Here's how the part is built. I have some questions about the finished solid (model axes, mm). Face numbers are marked on the shaded views. A direction names the side the tool comes from. Round coordinates to 2 decimals unless told otherwise and drop trailing zeros. Write each loop counter-clockwise with the first axis right and the second up, starting at its lowest first coordinate (ties: lowest second). Pieces come first, ordered by that corner, then holes. Notation, with made-up numbers: M -7.75,-32 L 20.25,-32 A14 cw 20.25,-12 Z; hole C 56.5,47.25 d5. An arc over 180 degrees is marked long. Write item = value, one per line. Start each with the question number.
(1) I need wall thicknesses on line 1 along X through (y, z) = (34, 38); line 2 along X through (y, z) = (-4, 9); line 3 along X through (y, z) = (-7.5, 22). Which ranges of each line are inside material? Lowest first, please.
(2) Will these pins go through, and if not, where does the flat tip stop? pin 1 Ø1.6 at (x, z) = (-6.5, -9) entering from -Y; pin 2 Ø3.5 at (x, z) = (-69, 12) entering from -Y; pin 3 Ø8 at (x, z) = (-47, 62) entering from -Y; pin 4 Ø11 at (y, z) = (8.5, -4.5) entering from -X.
(3) I want a section at A-A (z = 147.5). List the corners of the cut face in (x, y) for me.
(4) On a 3-axis mill with a long thin cutter (end or side, diameter ignored), from which of +Z, -Z, +X, -X, +Y, -Y can I reach the whole of each face in a straight line? I mean the marked faces 1 and 2. Say none if no direction works.
(5) I want a section at B-B (y = 44.5). List the corners of the cut face in (x, z) for me.
(6) I want a section at D-D (x = 31). List the corners of the cut face in (y, z) for me.
(7) I want a section at C-C (x = 75.5). List the corners of the cut face in (y, z) for me, and give its area (3 significant figures).
```python
from build123d import *

# Parameters (mm, degrees)
EXTRUDE_1_DEPTH          = 3
EXTRUDE_2_DEPTH          = 121.210911
SKETCH_3_W               = 47.605950515
SKETCH_3_H               = 3
CUT_EXTRUDE_1_DEPTH      = 99
SKETCH_5_W               = 185.441878516
SKETCH_5_H               = 108.742952173
CUT_EXTRUDE_2_DEPTH      = 1.5
SKETCH_6_W               = 175.21190103
SKETCH_6_H               = 36.65
EXTRUDE_3_DEPTH          = 7.2
SHELL_START              = 5.5
SHELL_1_DEPTH            = 114.710911355
SHELL_START_2            = 2.5
SHELL_1_2_OUTLINE_W      = 170.21190103
SHELL_1_2_OUTLINE_H      = 34.15
SHELL_1_2_DEPTH          = 124.910911355
SHELL_1_3_DEPTH          = 20.210911355
SHELL_1_4_DEPTH          = 17.210911355
SKETCH_7_W               = 170.21190103
SKETCH_7_H               = 34.15
CUT_EXTRUDE_3_DEPTH      = 7.2
SKETCH_8_W               = 2.5
SKETCH_8_H               = 36.65
EXTRUDE_4_DEPTH          = 45
CUT_EXTRUDE_4_DEPTH      = 261.975558395
SKETCH_10_W              = 2.5
SKETCH_10_H              = 2.880985124
EXTRUDE_5_DEPTH          = 124.689092
SKETCH_11_W              = 36.523943303
SKETCH_11_H              = 3
EXTRUDE_6_DEPTH          = 15
SKETCH_12_W              = 36.475357481
SKETCH_12_H              = 3.054288943
EXTRUDE_7_DEPTH          = 15
FILLET_1_R               = 25
SKETCH_13_W              = 43.927566906
SKETCH_13_H              = 9.945864205
EXTRUDE_8_DEPTH          = 8
CUT_EXTRUDE_5_DEPTH      = 219.603325421
SKETCH_15_W              = 43.927566906
SKETCH_15_H              = 9.945864205
EXTRUDE_9_DEPTH          = 2
SKETCH_17_W              = 27.673413216
SKETCH_17_H              = 3
EXTRUDE_10_DEPTH         = 12
RIB_1_REACH              = 263.024
SKETCH_18_WALL_W         = 539.179228978
SKETCH_18_WALL_H         = 3
MIRROR_5_COPY_1_REACH    = 263.024
MIRROR_5_COPY_1_SKETCH_W = 539.179228978
MIRROR_5_COPY_1_SKETCH_H = 3
RIB_2_REACH              = 175.005
SKETCH_19_WALL_W         = 366.464948776
SKETCH_19_WALL_H         = 3
MIRROR_7_COPY_1_REACH    = 175.005
MIRROR_7_COPY_1_SKETCH_W = 366.464948776
MIRROR_7_COPY_1_SKETCH_H = 3
RIB_3_REACH              = 153.018
SKETCH_20_WALL_W         = 334.972416452
SKETCH_20_WALL_H         = 3
EXTRUDE_11_DEPTH         = 20.47
CUT_EXTRUDE_6_DEPTH      = 264.412642976


# Read off the part's stored shape, not the designer's step: 抽壳1
with BuildPart() as part:
    # 草图1 → 凸台-拉伸1 (new body)
    with BuildSketch(Plane.XY):
        Polygon((-100, 0), (-60, 0), (-60, -3.3), (-100, -3.3), (-100, -23.3), (100, -23.3), (100, -3.3), (60, -3.3), (60, 0), (100, 0), (100, 39.5), (-100, 39.5), align=None)
    extrude(amount=EXTRUDE_1_DEPTH)

    # 草图2 → 凸台-拉伸2 (add)
    with BuildSketch(Plane.XY.offset(3)):
        Polygon((40, -48.15), (-40, -48.15), (-40, -0.15), (-87.605950515, -0.030985124), (-87.605950515, 39.5), (87.605950515, 39.5), (87.605950515, -0.030985124), (40, -0.15), align=None)
    extrude(amount=EXTRUDE_2_DEPTH)

    # 草图3 → 切除-拉伸1 (cut)
    with BuildSketch(Plane.XY.offset(124.210911355)):
        with Locations((63.802975258, 1.35)):
            Rectangle(SKETCH_3_W, SKETCH_3_H)
        with Locations((-63.802975258, 1.35)):
            Rectangle(SKETCH_3_W, SKETCH_3_H)
    extrude(amount=-CUT_EXTRUDE_1_DEPTH, mode=Mode.SUBTRACT)

    # 草图5 → 切除-拉伸2 (cut)
    with BuildSketch(Plane.XY.offset(124.210911355)):
        with Locations((-1.343781728, 1.77370169)):
            Rectangle(SKETCH_5_W, SKETCH_5_H)
    extrude(amount=-CUT_EXTRUDE_2_DEPTH, mode=Mode.SUBTRACT)

    # 草图6 → 凸台-拉伸3 (add)
    with BuildSketch(Plane.XY.offset(122.710911355)):
        with Locations((0, 21.175)):
            Rectangle(SKETCH_6_W, SKETCH_6_H)
    extrude(amount=EXTRUDE_3_DEPTH)

    # 抽壳1 outline → 抽壳1 (cut)
    with BuildSketch(Plane.XY.offset(SHELL_START)):
        Polygon((-85.105950515, 39.5), (-85.105950515, 5.35), (-37.5, 5.35), (-37.5, -45.65), (37.5, -45.65), (37.5, 5.35), (85.105950515, 5.35), (85.105950515, 39.5), align=None)
    extrude(amount=SHELL_1_DEPTH, mode=Mode.SUBTRACT)

    # Shell 1 2 outline → Shell 1 2 (cut)
    with BuildSketch(Plane.XY.offset(SHELL_START_2)):
        with Locations((0, 22.425)):
            Rectangle(SHELL_1_2_OUTLINE_W, SHELL_1_2_OUTLINE_H)
    extrude(amount=SHELL_1_2_DEPTH, mode=Mode.SUBTRACT)

    # Shell 1 3 outline → Shell 1 3 (cut)
    with BuildSketch(Plane.XY.offset(SHELL_START_2)):
        Polygon((-85.105950515, 5.35), (-85.105950515, 2.5), (-57.5, 2.5), (-57.5, 2.393757812), (-37.5, 2.343757812), (-37.5, -20.8), (37.5, -20.8), (37.5, 2.343757812), (57.5, 2.393757812), (57.5, 2.5), (85.105950515, 2.5), (85.105950515, 5.35), align=None)
    extrude(amount=SHELL_1_3_DEPTH, mode=Mode.SUBTRACT)

    # Shell 1 4 outline → Shell 1 4 (cut)
    with BuildSketch(Plane.XY.offset(SHELL_START)):
        Polygon((-85.105950515, 2.5), (-85.105950515, 2.462772689), (-57.5, 2.393757812), (-57.5, 2.5), align=None)
        Polygon((85.105950515, 2.462772689), (85.105950515, 2.5), (57.5, 2.5), (57.5, 2.393757812), align=None)
    extrude(amount=SHELL_1_4_DEPTH, mode=Mode.SUBTRACT)

    # 草图7 → 切除-拉伸3 (cut)
    with BuildSketch(Plane.XY.offset(129.910911355)):
        with Locations((0, 22.425)):
            Rectangle(SKETCH_7_W, SKETCH_7_H)
    extrude(amount=-CUT_EXTRUDE_3_DEPTH, mode=Mode.SUBTRACT)

    # 草图8 → 凸台-拉伸4 (add)
    with BuildSketch(Plane.XY.offset(129.910911355)):
        with Locations((86.355950515, 21.175)):
            Rectangle(SKETCH_8_W, SKETCH_8_H)
    extrude_4 = extrude(amount=EXTRUDE_4_DEPTH)

    # 镜向1: 凸台-拉伸4 across plane
    add(extrude_4.mirror(Plane(origin=(0, 0, 0), x_dir=(0, 0, 1), z_dir=(1, 0, 0))))

    # 草图9 → 切除-拉伸4 (cut, through all)
    with BuildSketch(Plane(origin=(87.605950515, 0, 0), x_dir=(0, 0, -1), z_dir=(1, 0, 0))):
        with BuildLine():
            ThreePointArc((-153.435169701, 14.152379613), (-157.269646082, 19.530454036), (-163.545332043, 21.590225708))
            Line((-163.545332043, 21.590225708), (-164.318099098, 21.561993734))
            Line((-164.318099098, 21.561993734), (-174.910911355, 21.175))
            Line((-174.910911355, 21.175), (-174.910911355, 2.85))
            Line((-174.910911355, 2.85), (-149.900003415, 2.85))
            Line((-149.900003415, 2.85), (-153.435169701, 14.152379613))
        make_face()
    extrude(amount=-CUT_EXTRUDE_4_DEPTH, mode=Mode.SUBTRACT)

    # 草图10 → 凸台-拉伸5 (add)
    with BuildSketch(Plane.XY.offset(25.210911355)):
        with Locations((86.355950515, 1.409507438)):
            Rectangle(SKETCH_10_W, SKETCH_10_H)
        with Locations((-86.355950515, 1.409507438)):
            Rectangle(SKETCH_10_W, SKETCH_10_H)
    extrude(amount=EXTRUDE_5_DEPTH)

    # 草图11 → 凸台-拉伸6 (add)
    with BuildSketch(Plane(origin=(40, 0, 0), x_dir=(0, 0, -1), z_dir=(1, 0, 0))):
        with Locations((-104.448939704, -4.8)):
            Rectangle(SKETCH_11_W, SKETCH_11_H)
    extrude_6 = extrude(amount=EXTRUDE_6_DEPTH)

    # 镜向2: 凸台-拉伸6 across plane
    add(extrude_6.mirror(Plane(origin=(0, 0, 0), x_dir=(0, 0, 1), z_dir=(1, 0, 0))))

    # 草图12 → 凸台-拉伸7 (add)
    with BuildSketch(Plane(origin=(40, 0, 0), x_dir=(0, 0, -1), z_dir=(1, 0, 0))):
        with Locations((-104.525351124, 1.496159348)):
            Rectangle(SKETCH_12_W, SKETCH_12_H)
    extrude_7 = extrude(amount=EXTRUDE_7_DEPTH)

    # 镜向3: 凸台-拉伸7 across plane
    add(extrude_7.mirror(Plane(origin=(0, 0, 0), x_dir=(0, 0, 1), z_dir=(1, 0, 0))))

    # 圆角1
    fillet_1_edges = [part.edges().sort_by_distance(p)[0] for p in [
        (0, -48.15, 122.710911355),
        (0, -45.65, 120.210911355),
    ]]
    fillet(fillet_1_edges, radius=FILLET_1_R)

    # 草图13 → 凸台-拉伸8 (add)
    with BuildSketch(Plane(origin=(0, 0, 0), x_dir=(-1, 0, 0), z_dir=(0, 0, -1))):
        with Locations((0, 10.69739906)):
            Rectangle(SKETCH_13_W, SKETCH_13_H)
    extrude(amount=EXTRUDE_8_DEPTH)

    # 草图14 → 切除-拉伸5 (cut, through all)
    with BuildSketch(Plane(origin=(21.963783453, 0, 0), x_dir=(0, 0, -1), z_dir=(1, 0, 0))):
        with BuildLine():
            add(Edge.make_bspline(
                [(0, 15.670331162), (4.03969355, 12.74473692), (8, 15.670331162)],
                knots=[0, 0, 0, 1, 1, 1], degree=2))
            Line((8, 15.670331162), (0, 15.670331162))
        make_face()
        with BuildLine():
            add(Edge.make_bspline(
                [(0, 5.724466957), (4.03969355, 8.650061199), (8, 5.724466957)],
                knots=[0, 0, 0, 1, 1, 1], degree=2))
            Line((8, 5.724466957), (0, 5.724466957))
        make_face()
    extrude(amount=-CUT_EXTRUDE_5_DEPTH, mode=Mode.SUBTRACT)

    # 草图15 → 凸台-拉伸9 (add)
    with BuildSketch(Plane(origin=(0, 0, -8), x_dir=(-1, 0, 0), z_dir=(0, 0, -1))):
        with Locations((0, 10.69739906)):
            Rectangle(SKETCH_15_W, SKETCH_15_H)
    extrude(amount=EXTRUDE_9_DEPTH)

    # 草图17 → 凸台-拉伸10 (add)
    with BuildSketch(Plane.XY.offset(3)):
        with Locations((73.836706608, -4.8)):
            Rectangle(SKETCH_17_W, SKETCH_17_H)
        with Locations((-73.836706608, -4.8)):
            Rectangle(SKETCH_17_W, SKETCH_17_H)
    extrude(amount=EXTRUDE_10_DEPTH)

    # 草图18 wall → 筋1 (add, up to next)
    with BuildSketch(Plane(origin=(87.673413216, -10.908430107, 9), x_dir=(0, -0.60913308834, -0.793068017694), z_dir=(0, 0.793068017694, -0.60913308834)), mode=Mode.PRIVATE) as rib_1_sk1:
        with Locations((0, 1.5)):
            Rectangle(SKETCH_18_WALL_W, SKETCH_18_WALL_H)
    rib_1_tool1 = extrude(rib_1_sk1.sketch, amount=RIB_1_REACH, mode=Mode.PRIVATE) - part.part
    rib_1 = rib_1_tool1.solids().sort_by_distance((87.673413216, -10.908430107, 9))[0]
    add(rib_1)

    # 镜向4: 筋1 across plane
    add(rib_1.mirror(Plane(origin=(73.836706608, 0, 0), x_dir=(0, 0, 1), z_dir=(1, 0, 0))))

    # 镜向5: 筋1 across plane
    add(rib_1.mirror(Plane(origin=(0, 0, 0), x_dir=(0, 0, 1), z_dir=(1, 0, 0))))

    # 镜向5 copy 1 sketch → 镜向5 copy 1 (add, up to next)
    with BuildSketch(Plane(origin=(-60, -10.908430107, 9), x_dir=(0, -0.60913308834, -0.793068017694), z_dir=(0, 0.793068017694, -0.60913308834)), mode=Mode.PRIVATE) as mirror_5_copy_1_sk1:
        with Locations((0, 1.5)):
            Rectangle(MIRROR_5_COPY_1_SKETCH_W, MIRROR_5_COPY_1_SKETCH_H)
    mirror_5_copy_1_tool1 = extrude(mirror_5_copy_1_sk1.sketch, amount=MIRROR_5_COPY_1_REACH, mode=Mode.PRIVATE) - part.part
    add(mirror_5_copy_1_tool1.solids().sort_by_distance((-60, -10.908430107, 9))[0])

    # 草图19 wall → 筋2 (add, up to next)
    with BuildSketch(Plane(origin=(47.5, -11.676129128, 122.710911355), x_dir=(-0.812759187769, -0.582599779176, 0), z_dir=(0.582599779176, -0.812759187769, 0)), mode=Mode.PRIVATE) as rib_2_sk1:
        with Locations((0, 1.5)):
            Rectangle(SKETCH_19_WALL_W, SKETCH_19_WALL_H)
    rib_2_tool1 = extrude(rib_2_sk1.sketch, amount=-RIB_2_REACH, mode=Mode.PRIVATE) - part.part
    rib_2 = rib_2_tool1.solids().sort_by_distance((47.5, -11.676129128, 122.710911355))[0]
    add(rib_2)

    # 镜向6: 筋2 across plane
    add(rib_2.mirror(Plane.XY.offset(104.448939704)))

    # 镜向7: 筋2 across plane
    add(rib_2.mirror(Plane(origin=(0, 0, 0), x_dir=(0, 0, 1), z_dir=(1, 0, 0))))

    # 镜向7 copy 1 sketch → 镜向7 copy 1 (add, up to next)
    with BuildSketch(Plane(origin=(-47.5, -11.676129128, 86.186968052), x_dir=(0.812759187769, -0.582599779176, 0), z_dir=(-0.582599779176, -0.812759187769, 0)), mode=Mode.PRIVATE) as mirror_7_copy_1_sk1:
        with Locations((0, 1.5)):
            Rectangle(MIRROR_7_COPY_1_SKETCH_W, MIRROR_7_COPY_1_SKETCH_H)
    mirror_7_copy_1_tool1 = extrude(mirror_7_copy_1_sk1.sketch, amount=-MIRROR_7_COPY_1_REACH, mode=Mode.PRIVATE) - part.part
    add(mirror_7_copy_1_tool1.solids().sort_by_distance((-47.5, -11.676129128, 86.186968052))[0])

    # 草图20 wall → 筋3 (add, up to next)
    with BuildSketch(Plane(origin=(75.091649782, 17.139028744, 72.5), x_dir=(-0.647409171989, -0.762142613967, 0), z_dir=(0.762142613967, -0.647409171989, 0)), mode=Mode.PRIVATE) as rib_3_sk1:
        Rectangle(SKETCH_20_WALL_W, SKETCH_20_WALL_H)
    rib_3_tool1 = extrude(rib_3_sk1.sketch, amount=RIB_3_REACH, mode=Mode.PRIVATE) - part.part
    rib_3 = rib_3_tool1.solids().sort_by_distance((75.091649782, 17.139028744, 72.5))[0]
    add(rib_3)

    # 镜向8: 筋3 across plane
    add(rib_3.mirror(Plane(origin=(0, 0, 0), x_dir=(0, 0, 1), z_dir=(1, 0, 0))))

    # 草图21 → 凸台-拉伸11 (add)
    with BuildSketch(Plane(origin=(0, 39.5, 0), x_dir=(1, 0, 0), z_dir=(0, 1, 0))):
        Polygon((-87.605950515, -174.910911355), (-85.105950515, -174.910911355), (-85.105950515, -2.5), (85.105950515, -2.5), (85.105950515, -174.910911355), (87.605950515, -174.910911355), (87.605950515, -3), (100, -3), (100, 0), (87.605950515, 0), (85.105950515, 0), (-85.105950515, 0), (-87.605950515, 0), (-100, 0), (-100, -3), (-87.605950515, -3), align=None)
    extrude(amount=EXTRUDE_11_DEPTH)

    # 草图22 → 切除-拉伸6 (cut, through all)
    with BuildSketch(Plane(origin=(87.605950515, 0, 0), x_dir=(0, 0, -1), z_dir=(1, 0, 0))):
        with BuildLine():
            Line((-149.900003415, -0.030985124), (-149.900003415, 24.969014876))
            ThreePointArc((-149.900003415, 24.969014876), (-152.828935603, 32.040082688), (-159.900003415, 34.969014876))
            Line((-159.900003415, 34.969014876), (-174.910911355, 34.969014876))
            Line((-174.910911355, 34.969014876), (-174.910911355, -0.030985124))
            Line((-174.910911355, -0.030985124), (-149.900003415, -0.030985124))
        make_face()
    extrude(amount=-CUT_EXTRUDE_6_DEPTH, mode=Mode.SUBTRACT)


solid = part.part
```
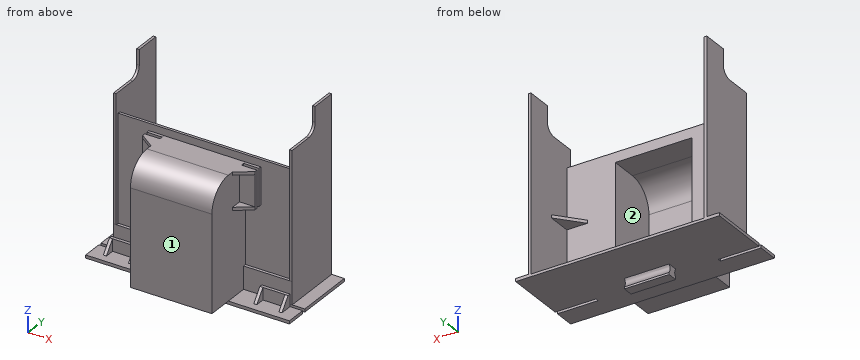
Returned:
q1.line_1 = -87.61 to -85.11, 85.11 to 87.61
q1.line_2 = -87.67 to -60, -40 to -37.5, 37.5 to 40, 60 to 87.67
q1.line_3 = -40 to -37.5, 37.5 to 40
q2.pin_1 = 5.72
q2.pin_2 = -6.3
q2.pin_3 = 2.85
q2.pin_4 = -100
q3.outline = M -87.61,-0.03 L -85.11,-0.03 L -85.11,59.97 L -87.61,59.97 Z; M 85.11,-0.03 L 87.61,-0.03 L 87.61,59.97 L 85.11,59.97 Z
q4.face_1 = +Z, -Z, +X, -X, -Y
q4.face_2 = +Y
q5.outline = M -100,0 L 100,0 L 100,3 L 87.61,3 L 87.61,174.91 L 85.11,174.91 L 85.11,2.5 L -85.11,2.5 L -85.11,174.91 L -87.61,174.91 L -87.61,3 L -100,3 Z
q6.outline = M -48.15,3 L -23.3,3 L -23.3,0 L 59.97,0 L 59.97,2.5 L -20.8,2.5 L -20.8,5.5 L -45.65,5.5 L -45.65,95.21 A25 cw -20.65,120.21 L 5.35,120.21 L 5.35,129.91 L 2.85,129.91 L 2.85,122.71 L -23.15,122.71 A25 ccw -48.15,97.71 Z
q7.outline = M -23.3,0 L -3.3,0 L -3.3,15 L -6.3,15 L -6.3,3 L -23.3,3 Z; M -0.06,3 L 0,3 L 0,0 L 59.97,0 L 59.97,2.5 L 2.5,2.5 L 2.5,5.5 L 2.44,5.5 L 2.44,22.71 L 5.35,22.71 L 5.35,71 L 17.62,71 L 17.62,74 L 5.35,74 L 5.35,129.91 L 2.85,129.91 L 2.85,25.21 L -0.06,25.21 Z
q7.area = 609 mm²
